Here's how the part is built. I have some questions about the finished solid (model axes, mm). Face numbers are marked on the shaded views. A direction names the side the tool comes from. Round coordinates to 2 decimals unless told otherwise and drop trailing zeros. Order: outer loops, then holes, each group sorted by start corner. A loop starts at its lowest first (then second) coordinate and runs counter-clockwise, first axis right, second up. Notation, with made-up numbers: (72, 57.5) -> (100, 57.5) arc R22 ccw to (100, 69.5) -> close; hole circle Ø11 at (77, -4). An arc over 180 degrees is marked (long way). Use a Markdown table: item, result. Add a question column.
(1) I want a section at C-C, the plane y = -110. Please give me the cut outline in (x, z), then the cut area to 3 significant figures.
(2) I want a section at A-A, the plane y = -68. Please give me the cut outline in (x, z), then the cut area to 3 significant figures.
(3) I'm going to push flat-ended pins straight in: P1, Ø7, axis at y = -68, z = 0, coming from the +X side; P2, Ø5.5, axis at x = -11, z = 0, coming from the +Y side; P3, Ø12, axis at x = 6.5, y = -84.5, coming from the +Z side; P4, Ø5.5, axis at x = 11, z = 3.5, coming from the +Y side. Where does each tip first touch, or does it pass through?
(4) I want a section at B-B, the plane y = -170. Please give me the cut outline in (x, z).
(5) I want a section at D-D, the plane x = 10.5. Please give me the cut outline in (y, z), then the cut area to 3 significant figures.
(6) On a 3-axis mill with a long thin cutter (end or side, diameter ignored), from which of +Z, -Z, +X, -X, +Y, -Y can I reach the whole of each face in a straight line? I mean the marked faces 1, 2 and 3. Say none if no direction works.
(7) If I drill on probe 1 along Y at (x, z) = (0.5, 0); probe 2 along Y at (x, z) = (-2.75, 0); probe 3 along Z at (x, y) = (0, -176), over which ranges is the centre line in solid material (lowest first)?
from build123d import *

# Parameters (mm, degrees)
F0_R          = 12.5
F1_DEPTH      = 190
F3_D          = 10
F3_DEPTH      = 26
F3_TIP        = 3.0043030951
F4_R          = 4.25
F5_DEPTH      = 25
F5_DEPTH_BACK = 25
F7_W          = 101
F7_H          = 25
F8_DEPTH      = 5
F10_W         = 163
F10_H         = 25
F11_DEPTH     = 5


with BuildPart() as f1:
    # F0 (on Front) → F1 (new body)
    with BuildSketch(Plane.XZ):
        Circle(F0_R)
    extrude(amount=F1_DEPTH)

    # F3
    with Locations(Plane.XZ.offset(190)):
        with Locations((0, 0)):
            Hole(F3_D / 2, depth=F3_DEPTH)
            with Locations((0, 0, -(F3_DEPTH + F3_TIP / 2))):  # 118° drill point
                Cone(0, F3_D / 2, F3_TIP, mode=Mode.SUBTRACT)

    # F4 (on Right) → F5 (cut, two sides)
    with BuildSketch(Plane.YZ) as f5_sk:
        with Locations((-18, 0)):
            Circle(F4_R)
        with Locations((-68, 0)):
            Circle(F4_R)
    extrude(amount=-F5_DEPTH, mode=Mode.SUBTRACT)
    extrude(f5_sk.sketch, amount=F5_DEPTH_BACK, mode=Mode.SUBTRACT)

    # F7 (on offset) → F8 (cut)
    with BuildSketch(Plane.YZ.offset(-12.5)):
        with Locations((-50.5, 0)):
            Rectangle(F7_W, F7_H)
    extrude(amount=F8_DEPTH, mode=Mode.SUBTRACT)

    # F10 (on offset) → F11 (cut)
    with BuildSketch(Plane.YZ.offset(12.5)):
        with Locations((-81.5, 0)):
            Rectangle(F10_W, F10_H)
    extrude(amount=-F11_DEPTH, mode=Mode.SUBTRACT)


solid = f1.part
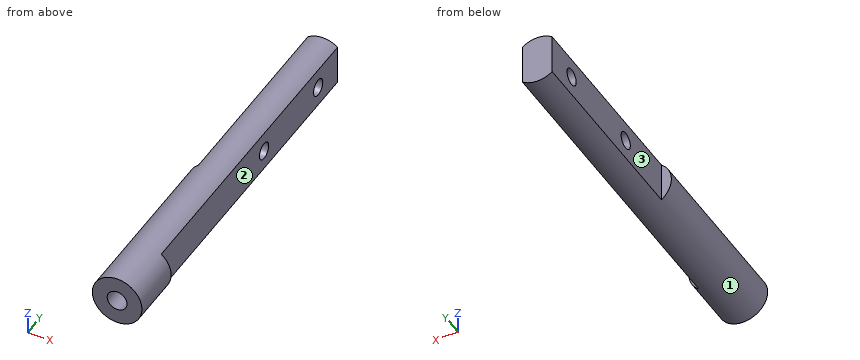
Taken from the geometry:
| question | item | result |
|---|---|---|
| 1 | outline | (7.5, -10) -> (7.5, 10) arc R12.5 ccw (long way) to start |
| 1 | area | 421 mm2 |
| 2 | outline | (-7.5, -10) arc R12.5 ccw to (7.5, -10) -> (7.5, -4.25) -> (-7.5, -4.25) -> close; (-7.5, 4.25) -> (7.5, 4.25) -> (7.5, 10) arc R12.5 ccw to (-7.5, 10) -> close |
| 2 | area | 224 mm2 |
| 3 | P1 | passes through |
| 3 | P2 | stops at y = -101 |
| 3 | P3 | stops at z = 12.49 |
| 3 | P4 | stops at y = -163 |
| 4 | outline | circle Ø25 at (0, 0); hole circle Ø10 at (0, 0) |
| 5 | outline | (-190, -6.78) -> (-163, -6.78) -> (-163, 6.78) -> (-190, 6.78) -> close |
| 5 | area | 366 mm2 |
| 6 | face 1 | +Y, -Y |
| 6 | face 2 | +Z, -Z, +X, +Y |
| 6 | face 3 | +Z, -Z, -X, +Y |
| 7 | probe 1 | y = -161.3 to -72.25, -63.75 to -22.25, -13.75 to 0 |
| 7 | probe 2 | y = -162.65 to -72.25, -63.75 to -22.25, -13.75 to 0 |
| 7 | probe 3 | z = -12.5 to -5, 5 to 12.5 |
